Geometry: final body of the model. Coordinates: model frame, mm. Round coordinates to 2 decimals unless told otherwise and drop trailing zeros. Loops run counter-clockwise (first coordinate to the right, second up) from the corner with the lowest first, then second, coordinate; pieces in that order, holes last. Notation, with made-up numbers: (0, 76.5) - (12, 76.5) arc R25 ccw to (12, 97.5) - close; hole circle Ø10 at (-16.5, -5). An arc over 180 degrees is marked (long way). Write item = value, one per line. Start each with the question number.
Item 1: Draft query along Z for faces 1 (the cylindrical face through (-3.797, 5.07, -58.859)), 2 (the cylindrical face through (-3.859, 5.07, 58.797)), 3 (the cylindrical face through (-0.676, 4.93, 17.146)). Return one class per face: pulls with the +Z half, pulls with the -Z half, needs draft (parallel to the pull), parting line crosses it, or undercut.
Item 2: Section C-C (z = -34.5). Return loops of the section in (x, y).
Item 3: Line query: line 1 (X direction, y = 4.5, z = 15); line 2 (X direction, y = 1.5, z = -17); line 3 (Z direction, x = 4, y = 9.5). Output: solid intervals per line, ascending. Write a range as from..to.
Item 4: First-contact query: pin 1 (4 mm diameter, centred on x = 3.5, y = 2, fed in from +Z). Flat tip, straight axial feed; report the tip coordinate or a pass-through.
Item 5: Section B-B (y = 8). Count the separate pieces of the cut face and the enclosed holes in it, plus the area to 3 significant figures.
Item 6: Section A-A (z = 45). Return loops of the section in (x, y).
Autodesk Inventor part; units mm, degrees
ref_plane "YZ Plane" through (0, 0, 0) normal (1, 0, 0) x (0, 1, 0)
ref_plane "XZ Plane" through (0, 0, 0) normal (0, 1, 0) x (-1, 0, 0)
ref_plane "XY Plane" through (0, 0, 0) normal (0, 0, 1) x (1, 0, 0)
sketch "Sketch1" plane through (0, 0, 0) normal (0, 1, 0) x (-1, 0, 0)
  line L0 (5, 60) -> (-5, 60)
  line L1 (-5, 60) -> (-5, -60)
  line L2 (-5, -60) -> (5, -60)
  line L3 (5, -60) -> (5, 60)
  line L4 (5, 60) -> (-5, -60) construction
  line L5 (-5, 60) -> (5, -60) construction
  point P0 (0, 0)
  dimension "d0" = 10
  dimension "d1" = 120
extrude "Extrusion1" add sketch "Sketch1" along normal blind 10
fillet "Fillet1" radius 4 4 edges at (5, 5, 60) (-5, 5, 60) (-5, 5, -60) (5, 5, -60)
sketch "Sketch2" plane through (0, 10, 0) normal (0, 1, 0) x (1, 0, 0)
  line L0 (1, 60) -> (-1, 60)
  line L1 (0, 60) -> (0, -50)
  line L2 (-1, 60) -> (-1, 55)
  arc A0 (-1, 60) -> (-5, 56) centre (-1, 56) ccw
  line L3 (-1, 55) -> (0, 55)
  point P0 (0, 0)
  dimension "d5" = 110
  dimension "d6" = 5
hole "Hole1" at (0, 10, -55) direction (0, -1, 0) diameter 4.5 depth 12
pattern_linear "Rectangular Pattern1" count 12 spacing 10 along (0, 0, 1) of "Hole1"
properties part number "soporte de direccion2"
Taken from the geometry:
q1.face_1 = pulls with the -Z half
q1.face_2 = pulls with the +Z half
q1.face_3 = undercut
q2.outline = (-5, 0) - (-2.19, 0) - (-2.19, 10) - (-5, 10) - close; (2.19, 0) - (5, 0) - (5, 10) - (2.19, 10) - close
q3.line_1 = -5..-2.25, 2.25..5
q3.line_2 = -5..-1.03, 1.03..5
q3.line_3 = -58.65..58.65
q4.pin_1 = 59.97
q5.separate_pieces = 1
q5.enclosed_holes = 12
q5.area = 995 mm^2
q6.outline = (-5, 0) - (-2.25, 0) - (-2.25, 10) - (-5, 10) - close; (2.25, 0) - (5, 0) - (5, 10) - (2.25, 10) - close
